```python
from build123d import *

# Parameters (mm, degrees)
F0_W     = 228.6
F0_H     = 19.05
F0_R     = 2.9845
F1_DEPTH = 12.7
F2_DEPTH = 25.4
F3_R     = 2.9845
F4_DEPTH = 12.7
F5_R     = 9.52499


# Not quite as in the source:
# - a fillet or chamfer is up to 0.001 mm smaller than in the source, because OpenCascade refuses the exact size
# - a feature names something its author has since deleted; it is built from what else it names


with BuildPart() as f1:
    # F0 (on Front) → F1 (new body)
    with BuildSketch(Plane.XZ):
        with Locations((3.2032227146, 0)):
            Rectangle(F0_W, F0_H)
        with Locations((-101.6, 0)):
            Circle(F0_R, mode=Mode.SUBTRACT)
        with Locations((-76.2, 0)):
            Circle(F0_R, mode=Mode.SUBTRACT)
        with Locations((-50.8, 0)):
            Circle(F0_R, mode=Mode.SUBTRACT)
        with Locations((-25.4, 0)):
            Circle(F0_R, mode=Mode.SUBTRACT)
        Circle(F0_R, mode=Mode.SUBTRACT)
        with Locations((25.4, 0)):
            Circle(F0_R, mode=Mode.SUBTRACT)
        with Locations((50.8, 0)):
            Circle(F0_R, mode=Mode.SUBTRACT)
        with Locations((76.2, 0)):
            Circle(F0_R, mode=Mode.SUBTRACT)
        with Locations((101.6, 0)):
            Circle(F0_R, mode=Mode.SUBTRACT)
    extrude(amount=F1_DEPTH)

    # F0 (on Front) → F2 (join)
    with BuildSketch(Plane.XZ):
        Circle(F0_R)
        with Locations((-101.6, 0)):
            Circle(F0_R)
        with Locations((-76.2, 0)):
            Circle(F0_R)
        with Locations((-50.8, 0)):
            Circle(F0_R)
        with Locations((-25.4, 0)):
            Circle(F0_R)
        with Locations((25.4, 0)):
            Circle(F0_R)
        with Locations((50.8, 0)):
            Circle(F0_R)
        with Locations((76.2, 0)):
            Circle(F0_R)
        with Locations((101.6, 0)):
            Circle(F0_R)
    extrude(amount=F2_DEPTH)

    # F3 (on face) → F4 (join)
    with BuildSketch(Plane(origin=(0, 0, 0), x_dir=(-1, 0, 0), z_dir=(0, 1, 0))):
        with Locations((-76.2, 0)):
            Circle(F3_R)
    extrude(amount=F4_DEPTH)

    # F5 (radius 9.525 in the source; OpenCascade refuses exactly that, so slightly less here)
    f5_edges = [f1.edges().sort_by_distance(p)[0] for p in [
        (117.503223, -6.35, 9.525),
        (117.503223, -6.35, -9.525),
        (-111.096777, -6.35, 9.525),
        (-111.096777, -6.35, -9.525),
    ]]
    fillet(f5_edges, radius=F5_R)


solid = f1.part
```
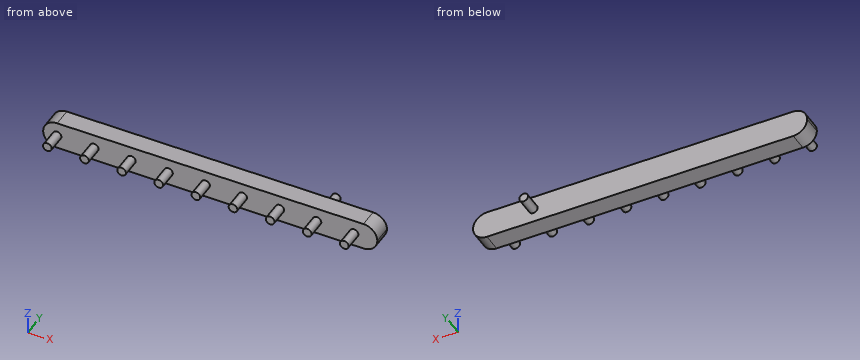
Model file for the job. Use its own axes, mm. Give positions to 0.01 mm unless a question says otherwise; leave off trailing zeros. Order: outer loops, then holes, each group sorted by start corner. A loop starts at its lowest first (then second) coordinate and runs counter-clockwise, first axis right, second up.
1) Saw through at B-B, the plane x = 76.2. Write the cut outline in (y, z) (1 decimal).
2) Saw through at C-C, the plane x = 0. Write the cut outline in (y, z) (1 decimal).
3) Pin check, flat tips, straight feed: pin 1 (6 mm diameter, centred on x = -61.5, z = -4, fed in from +Y); pin 2 (1.5 mm diameter, centred on y = -13.5, z = -1.5, fed in from +X); pin 3 (3 mm diameter, centred on x = -83, z = 6.5, fed in from -Y). Stop position of each tip, or through.
4) Wall check: probe 1 along Y at (x, z) = (62.5, -3.5); probe 2 along X at (y, z) = (6, 0.5); probe 3 along X at (y, z) = (-6, -6.75). Give the ranges that are in metal, low to high.
5) Saw through at D-D, the plane z = -6.5. Write the cut outline in (x, y).
Computed:
1. outline: (-25.4, -3) - (-12.7, -3) - (-12.7, -9.5) - (0, -9.5) - (0, -3) - (12.7, -3) - (12.7, 3) - (0, 3) - (0, 9.5) - (-12.7, 9.5) - (-12.7, 3) - (-25.4, 3) - close
2. outline: (-25.4, -3) - (-12.7, -3) - (-12.7, -9.5) - (0, -9.5) - (0, 9.5) - (-12.7, 9.5) - (-12.7, 3) - (-25.4, 3) - close
3. pin 1: stops at y = 0
3. pin 2: stops at x = 104.49
3. pin 3: stops at y = -12.7
4. probe 1: y = -12.7 to 0
4. probe 2: x = 73.26 to 79.14
4. probe 3: x = -108.29 to 114.7
5. outline: (-108.53, -12.7) - (114.94, -12.7) - (114.94, 0) - (-108.53, 0) - close
